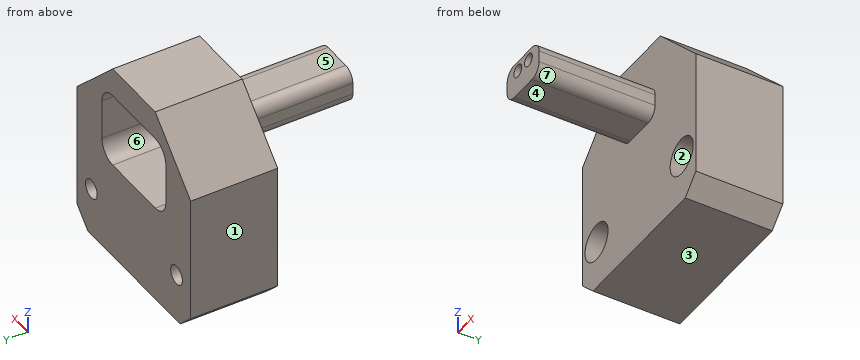
```python
from build123d import *

# Parameters (mm, degrees)
F1_DEPTH       = 15
F2_W           = 9
F2_H           = 6
F3_DEPTH       = 20
F4_W           = 18
F4_H           = 13
F5_DEPTH       = 13
F6_R           = 3
F7_D           = 3.3
F7_CBORE_D     = 6.5
F7_CBORE_DEPTH = 6
F9_D           = 1.76
F9_CBORE_D     = 2.2
F9_CBORE_DEPTH = 13
F10_R          = 2


with BuildPart() as f1:
    # F0 (on Front) → F1 (new body)
    with BuildSketch(Plane.XZ):
        Polygon((22, 0), (10, 0), (0, -10), (0, -32), (3, -35), (29, -35), (32, -32), (32, -10), align=None)
    extrude(amount=F1_DEPTH)

    # F2 (on face) → F3 (join)
    with BuildSketch(Plane.XZ.offset(15)):
        with Locations((16, -11)):
            Rectangle(F2_W, F2_H)
    extrude(amount=F3_DEPTH)

    # F4 (on face) → F5 (cut)
    with BuildSketch(Plane(origin=(0, 0, 0), x_dir=(-1, 0, 0), z_dir=(0, 1, 0))):
        with Locations((-16, -11.5)):
            Rectangle(F4_W, F4_H)
    extrude(amount=-F5_DEPTH, mode=Mode.SUBTRACT)

    # F6
    f6_edges = [f1.edges().sort_by_distance(p)[0] for p in [
        (25, -6.5, -5),
        (7, -6.5, -5),
        (25, -6.5, -18),
        (7, -6.5, -18),
    ]]
    fillet(f6_edges, radius=F6_R)

    # F7 (through all)
    with Locations(Plane.XZ.offset(15)):
        with Locations((4, -26.5), (28, -26.5)):
            CounterBoreHole(F7_D / 2, F7_CBORE_D / 2, F7_CBORE_DEPTH)

    # F9 (through all)
    with Locations(Plane.XZ.offset(35)):
        with Locations((14.5, -9.7), (17.5, -9.7)):
            CounterBoreHole(F9_D / 2, F9_CBORE_D / 2, F9_CBORE_DEPTH)

    # F10
    f10_edges = [f1.edges().sort_by_distance(p)[0] for p in [
        (20.5, -25, -8),
        (20.5, -25, -14),
        (11.5, -25, -8),
        (11.5, -25, -14),
    ]]
    fillet(f10_edges, radius=F10_R)


solid = f1.part
```
Check sheet for the modelled part. Datum: model origin and axes. Units: mm. Face numbers are marked on the shaded views. A direction names the side the tool comes from. Coordinates: 2 decimals unless noted, no trailing zeros. Loops run counter-clockwise (first coordinate to the right, second up) from the corner with the lowest first, then second, coordinate; pieces in that order, holes last.
1) Gauge pin test, flat ends, axial feed: pin 1 (5.5 mm diameter, centred on x = 28, z = -26.5, fed in from -Y); pin 2 (2.5 mm diameter, centred on x = 18, z = -9.5, fed in from -Y); pin 3 (5 mm diameter, centred on y = -5, z = -7, fed in from -X); pin 4 (2 mm diameter, centred on y = -28, z = -11, fed in from +X). Record the tip position at first contact, or that the pin passes through.
2) Sectioned sample at B-B (z = -26.5). Record the boundary of the cut face in (x, y).
3) Access from +Z, -Z, +X, -X, +Y, -Y to the whole of each face (thin tool, end or side, straight path). Record for the marked faces 4, 5, 6 and 7.
4) Material ranges on probe 1 along Z at (x, y) = (14.5, -28); probe 2 along Z at (x, y) = (20, -12.5); probe 3 along Y at (x, z) = (5, -13), recorded low to high.
5) Sectioned sample at C-C (y = -3.5). Record the boundary of the cut face in (x, z), and give its area (3 significant figures).
6) Sectioned sample at D-D (x = 17.5). Record the boundary of the cut face in (y, z), and give its area (3 significant figures).
7) Release check for a two-part mould opening along X. For the marked faces 1, 2 and 3 record: released by +X, released by -X, zero draft, split by the parting line, or undercut.
8) Sectioned sample at A-A (x = 28). Record the boundary of the cut face in (y, z).
Check sheet entries:
1. pin 1: stops at y = -9
1. pin 2: stops at y = -35
1. pin 3: stops at x = 0.5
1. pin 4: stops at x = 20.5
2. outline: (0, -15) - (0.75, -15) - (0.75, -9) - (2.35, -9) - (2.35, 0) - (0, 0) - close; (5.65, -9) - (7.25, -9) - (7.25, -15) - (24.75, -15) - (24.75, -9) - (26.35, -9) - (26.35, 0) - (5.65, 0) - close; (29.65, -9) - (31.25, -9) - (31.25, -15) - (32, -15) - (32, 0) - (29.65, 0) - close
3. face 4: -Z, +X, -X, -Y
3. face 5: +Z, +X, -X, -Y
3. face 6: +Y
3. face 7: -Z, +X, -Y
4. probe 1: z = -14 to -10.8, -8.6 to -8
4. probe 2: z = -35 to -18, -5 to 0
4. probe 3: y = -15 to 0
5. outline: (0, -32) - (3, -35) - (29, -35) - (32, -32) - (32, -10) - (22, 0) - (10, 0) - (0, -10) - close; hole circle Ø3.3 at (4, -26.5); hole (7, -15) arc R3 ccw to (10, -18) - (22, -18) arc R3 ccw to (25, -15) - (25, -8) arc R3 ccw to (22, -5) - (10, -5) arc R3 ccw to (7, -8) - close; hole circle Ø3.3 at (28, -26.5)
5. area: 768 mm2
6. outline: (-35, -14) - (-15, -14) - (-15, -35) - (0, -35) - (0, -18) - (-13, -18) - (-13, -10.58) - (-22, -10.58) - (-22, -10.8) - (-35, -10.8) - close; (-35, -8.6) - (-22, -8.6) - (-22, -8.82) - (-13, -8.82) - (-13, -5) - (0, -5) - (0, 0) - (-15, 0) - (-15, -8) - (-35, -8) - close
6. area: 432 mm2
7. face 1: released by -X
7. face 2: undercut
7. face 3: zero draft
8. outline: (-15, -35) - (0, -35) - (0, -28.15) - (-9, -28.15) - (-9, -29.75) - (-15, -29.75) - close; (-15, -23.25) - (-9, -23.25) - (-9, -24.85) - (0, -24.85) - (0, -6) - (-15, -6) - close
